Geometry check sheet. Reference: the model listing, model coordinates, mm. A direction names the side the tool comes from. Round coordinates to 2 decimals unless told otherwise and drop trailing zeros. Write each loop counter-clockwise with the first axis right and the second up, starting at its lowest first coordinate (ties: lowest second). Pieces come first, ordered by that corner, then holes. Notation, with made-up numbers: M 76,42 L 98,42 A36 ccw 98,81 Z; hole C 79.25,-5.75 d6. An arc over 180 degrees is marked long. Answer in a Markdown table with one row per item. Add a question column.
from build123d import *

# Parameters (mm, degrees)
F0_W     = 18.8
F0_H     = 12
F1_DEPTH = 11
F2_W     = 21.2
F2_H     = 14.8
F3_DEPTH = 2.3
F4_SIZE  = 1.8
F5_W     = 16.6
F5_H     = 10.2
F6_DEPTH = 4.5
F8_DEPTH = 25


with BuildPart() as f1:
    # F0 (on Front) → F1 (new body)
    with BuildSketch(Plane.XZ):
        with Locations((9.4, -6)):
            Rectangle(F0_W, F0_H)
    extrude(amount=F1_DEPTH)

    # F2 (on face) → F3 (join)
    with BuildSketch(Plane.XZ.offset(11)):
        with Locations((9.453604, -5.990063)):
            Rectangle(F2_W, F2_H)
    extrude(amount=F3_DEPTH)

    # F4
    f4_edges = [f1.edges().sort_by_distance(p)[0] for p in [
        (-1.146396, -13.3, -5.990063),
        (9.453604, -13.3, -13.390063),
        (20.053604, -13.3, -5.990063),
        (9.453604, -13.3, 1.409937),
    ]]
    chamfer(f4_edges, length=F4_SIZE)

    # F5 (on face) → F6 (join)
    with BuildSketch(Plane.XZ.offset(13.3)):
        with Locations((9.453604, -5.990063)):
            Rectangle(F5_W, F5_H)
    extrude(amount=F6_DEPTH)

    # F7 (on face) → F8 (cut)
    with BuildSketch(Plane(origin=(0, 0, -11.090063), x_dir=(1, 0, 0), z_dir=(0, 0, -1))):
        Polygon((1.153604, 17.8), (1.153604, 13.3), (5.163922, 17.8), align=None)
        Polygon((17.753604, 17.8), (5.163922, 17.8), (17.753604, 13.3), align=None)
    extrude(amount=-F8_DEPTH, mode=Mode.SUBTRACT)


solid = f1.part
Item 1: Gauge pin test, flat ends, axial feed: pin 1 Ø2 at (x, y) = (3.5, -6.5) entering from -Z; pin 2 Ø1.3 at (x, y) = (6.5, -16) entering from -Z; pin 3 Ø2 at (x, z) = (2, -5.5) entering from +Y; pin 4 Ø2 at (x, z) = (13.5, -1.5) entering from -Y. Record the tip position at first contact, or that the pin passes through.
Item 2: Section check A-A, the plane z = -1.5. Record the boundary of the cut face in (x, y), and give its area (3 significant figures).
Item 3: Scan lines: probe 1 along X at (y, z) = (-10.25, -2.5); probe 2 along Z at (x, y) = (6.5, -6); probe 3 along Y at (x, z) = (18, -2.5). Record each from-to range of solid material in increasing order. Write a range as from..to.
Item 4: Access from +Z, -Z, +X, -X, +Y, -Y to the whole of each face (thin tool, end or side, straight path). Record for faces 1 (the flat face through (8.8, -13.3, -11.4)), 2 (the flat face through (7, -15, -0.89)), 3 (the flat face through (0, -5, -6)), 4 (the flat face through (18.8, -5, -6)).
Item 5: Section check D-D, the plane x = 7.75. Record the boundary of the cut face in (y, z), and give its area (3 significant figures).
Item 6: Section check B-B, the plane x = 15.5. Record the boundary of the cut face in (y, z).
Item 7: Section check C-C, the plane y = -1.25. Record the boundary of the cut face in (x, z), and give its area (3 significant figures).
Result sheet:
| question | item | result |
|---|---|---|
| 1 | pin 1 | stops at z = -12 |
| 1 | pin 2 | stops at z = -11.09 |
| 1 | pin 3 | stops at y = 0 |
| 1 | pin 4 | stops at y = -15.18 |
| 2 | outline | M -1.15,-11.5 L 0.65,-13.3 L 1.15,-13.3 L 5.16,-17.8 L 17.75,-13.3 L 18.25,-13.3 L 20.05,-11.5 L 20.05,-11 L 18.8,-11 L 18.8,0 L 0,0 L 0,-11 L -1.15,-11 Z |
| 2 | area | 290 mm^2 |
| 3 | probe 1 | x = 0..18.8 |
| 3 | probe 2 | z = -12..0 |
| 3 | probe 3 | y = -13.3..0 |
| 4 | face 1 | -Y |
| 4 | face 2 | +Z, +X, -X, -Y |
| 4 | face 3 | +Z, -Z, -X, +Y |
| 4 | face 4 | +Z, -Z, +X, +Y |
| 5 | outline | M -16.88,-11.09 L -13.3,-11.09 L -13.3,-11.59 L -11.5,-13.39 L -11,-13.39 L -11,-12 L 0,-12 L 0,0 L -11,0 L -11,1.41 L -11.5,1.41 L -13.3,-0.39 L -13.3,-0.89 L -16.88,-0.89 Z |
| 5 | area | 199 mm^2 |
| 6 | outline | M -14.11,-11.09 L -13.3,-11.09 L -13.3,-11.59 L -11.5,-13.39 L -11,-13.39 L -11,-12 L 0,-12 L 0,0 L -11,0 L -11,1.41 L -11.5,1.41 L -13.3,-0.39 L -13.3,-0.89 L -14.11,-0.89 Z |
| 7 | outline | M 0,-12 L 18.8,-12 L 18.8,0 L 0,0 Z |
| 7 | area | 226 mm^2 |
